Could you check a few things on this model? Use its own coordinates, in mm. A direction names the side the tool comes from. Give positions to 0.01 mm unless a question says otherwise; leave off trailing zeros. Loops run counter-clockwise (first coordinate to the right, second up) from the corner with the lowest first, then second, coordinate; pieces in that order, holes last. Notation, with made-up numbers: (15, 23) -> (32, 23) arc R20 cw to (32, 52) -> close; hole circle Ø1 at (49.25, 12.5). An arc over 180 degrees is marked (long way). Write each question's results on one line, items separated by ' | '. Start each with the question number.
Q1. If I drill on line 1 along X through (y, z) = (90, 38.5); line 2 along X through (y, z) = (82, 12); line 3 along Y through (x, z) = (44.5, 36), over which ranges is the centre line in solid material (lowest first)?
Q2. Which directions (+Z, -Z, +X, -X, +Y, -Y) give clear straight access to the entire face, cutting with the end or side of a thin tool? Please do faces 1 (the face through (-48.87, 88.85, 46.99)), 2 (the face through (-15.19, 85.274, 46.993)), 3 (the face through (12.503, 87.306, 19.72)).
Q3. Will these pins go through, and if not, where does the flat tip stop? P1, Ø2, axis at x = -29, z = 19, coming from the -Y side; P2, Ø6, axis at y = 32.5, z = 22, coming from the +X side; P3, Ø6, axis at y = 65, z = 11.5, coming from the -X side.
Q4. If we section it at A-A, the plane z = 32: List the corners of the cut face in (x, y) for me.
Q5. We'd pull the mould along X, two halves only. Please class faces 4 (the face through (-37.4, 41.465, 19.72)), 5 (the face through (15.078, 85.819, 46.993)), 6 (the face through (32.15, 102.29, 20.28)), 7 (the face through (-0.19, 5.15, 20.28)): released by +X, released by -X, zero draft, split by the parting line, or undercut.
from build123d import *

# Parameters (mm, degrees)
BOSS_EXTRUDE1_DEPTH = 50
FILLET1_R           = 10


with BuildPart() as part:
    # Sketch1 → Boss-Extrude1 (new body)
    with BuildSketch(Plane.XY):
        Polygon((0, 0), (-68.020648891, 75.4139), (-34.010324446, 106.09), (0, 75.4139), (32.252675554, 106.09), (64.505351109, 75.4139), align=None)
    extrude(amount=BOSS_EXTRUDE1_DEPTH)

    # Fillet1
    fillet1_edges = [part.edges().sort_by_distance(p)[0] for p in [
        (0, 0, 25),
        (32.252675554, 106.09, 25),
        (64.505351109, 75.4139, 25),
        (16.126337777, 90.75195, 50),
        (-17.005162223, 90.75195, 50),
        (-51.015486668, 90.75195, 50),
        (-34.010324446, 37.70695, 50),
        (32.252675554, 37.70695, 50),
        (48.379013332, 90.75195, 50),
    ]]
    fillet(fillet1_edges, radius=FILLET1_R)


solid = part.part
Final values:
1) line 1: x = -51.85 to -16.17, 15.34 to 49.17 | line 2: x = -60.72 to -7.3, 6.92 to 57.58 | line 3: y = 52.03 to 94.44
2) face 1: +Z, -X, +Y | face 2: +Z, +Y | face 3: +Z, -Z, +Y
3) P1: stops at y = 31.04 | P2: stops at x = 30.36 | P3: stops at x = -61.33
4) outline: (-68.02, 75.41) -> (-7.62, 8.45) arc R10 ccw to (7.4, 8.65) -> (58.34, 68.21) arc R10 ccw to (57.63, 81.95) -> (39.14, 99.54) arc R10 ccw to (25.36, 99.54) -> (0, 75.41) -> (-34.01, 106.09) -> close
5) face 4: released by -X | face 5: undercut | face 6: undercut | face 7: split by the parting line
